The listing builds one solid part. Answer for the finished solid, in the listing's coordinates (mm). Round coordinates to 2 decimals unless told otherwise and drop trailing zeros. Order: outer loops, then holes, each group sorted by start corner. A loop starts at its lowest first (then second) coordinate and runs counter-clockwise, first axis right, second up. Notation, with made-up numbers: (15.25, 86.25) -> (72.25, 86.25) arc R9 ccw to (72.25, 98.25) -> close; hole circle Ø1 at (18, 57). An arc over 180 degrees is marked (long way). Answer in a Markdown table with one row per item. Add a question column.
```python
from build123d import *

# Parameters (mm, degrees)
F1_DEPTH = 10


# Not quite as in the source:
# - a feature names something its author has since deleted; it is built from what else it names


with BuildPart() as f1:
    # F0 (on Front) → F1 (new body)
    with BuildSketch(Plane.XZ):
        Polygon((260, -100), (260, -110), (280, -110), (280, -100), (300, -100), (300, -110), (320, -110), (320, -100), (340, -100), (340, -110), (360, -110), (360, -100), (380, -100), (320, 40), (315.7142857143, 50), (300, 50), (300, 40), (280, 40), (280, 50), (260, 50), (260, 40), (250, 40), (250, 20), (260, 20), (260, 0), (250, 0), (250, -20), (260, -20), (260, -40), (250, -40), (250, -60), (260, -60), (260, -80), (250, -80), (250, -100), align=None)
    extrude(amount=-F1_DEPTH)


solid = f1.part
```
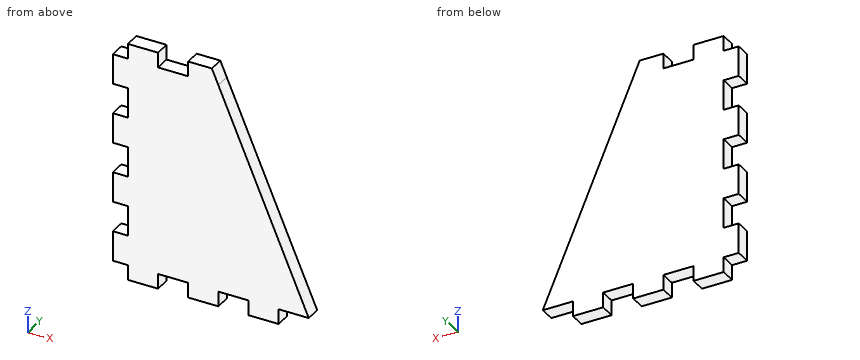
Item 1: Find the intervals of material crossed by probe 1 along Z at (x, y) = (287, 5.5); probe 2 along X at (y, z) = (3, -37); probe 3 along X at (y, z) = (8.25, -96.5), in increasing order. Write a range as [from, to].
Item 2: The part is cut by section A-A, the plane z = 8.5. Give the vertices of the cut face in (x, y).
Item 3: The part is cut by section B-B, the plane x = 344. Give the vertices of the cut face in (y, z), and give its area (3 significant figures).
Item 4: Flat-ended cylindrical pins translate along their axes: P1, Ø5, axis at y = 6.5, z = -72, coming from the -X side; P2, Ø5, axis at x = 297, y = 5, coming from the -Z side; P3, Ø5, axis at x = 255.5, y = 6.5, coming from the +Z side. Find the tip coordinate at first contact, or state that the pin passes through.
Resolved:
| question | item | result |
|---|---|---|
| 1 | probe 1 | [-100, 40] |
| 1 | probe 2 | [260, 353] |
| 1 | probe 3 | [250, 378.5] |
| 2 | outline | (260, 0) -> (333.5, 0) -> (333.5, 10) -> (260, 10) -> close |
| 3 | outline | (0, -110) -> (10, -110) -> (10, -16) -> (0, -16) -> close |
| 3 | area | 940 mm2 |
| 4 | P1 | x = 260 |
| 4 | P2 | z = -100 |
| 4 | P3 | z = 40 |
